from build123d import *

# Parameters (mm, degrees)
SKETCH1_W                    = 117.475
SKETCH1_H                    = 65.3161
BASE_FLANGE1_DEPTH           = 3.2639
F_10_0_1935_DIAMETER_HOLE1_D = 4.9149
BOSS_EXTRUDE1_DEPTH          = 3.2639
F_1_4_START                  = -3.2639
F_1_4_CLEARANCE_SLOT1_DEPTH  = 3.2639
F_10_0_1935_DIAMETER_HOLE2_D = 4.9149
FILLET1_R                    = 6.35
FILLET2_R                    = 12.7


# Read off the part's stored shape, not the designer's step: 1/4 Clearance Slot1
# Sheet-metal steps are written as plain solids
with BuildPart() as part:
    # Sketch1 → Base-Flange1 (new body)
    with BuildSketch(Plane.XY):
        with Locations((58.7375, 0)):
            Rectangle(SKETCH1_W, SKETCH1_H)
    extrude(amount=-BASE_FLANGE1_DEPTH)

    # #10 (0.1935) Diameter Hole1 (through all)
    with Locations(Plane.XY):
        with Locations((28.575, 19.05), (28.575, -19.05), (104.775, 19.05), (104.775, -19.05)):
            Hole(F_10_0_1935_DIAMETER_HOLE1_D / 2)

    # Sketch8 → Boss-Extrude1 (add)
    with BuildSketch(Plane.XY):
        Polygon((0, 32.65805), (-116.888396133, -111.687098016), (-55.202435442, -161.639404056), (49.244605652, -32.65805), (0, -32.65805), align=None)
    extrude(amount=-BOSS_EXTRUDE1_DEPTH)

    # 1/4 Clearance Slot1 outline → 1/4 Clearance Slot1 (cut)
    with BuildSketch(Plane.XY.offset(F_1_4_START)):
        with BuildLine():
            Line((-71.825899608, -91.951886399), (-67.506895384, -95.449347058))
            ThreePointArc((-67.506895384, -95.449347058), (-62.484066487, -94.921426468), (-63.011987077, -89.898597571))
            Line((-63.011987077, -89.898597571), (-67.330991301, -86.401136912))
            ThreePointArc((-67.330991301, -86.401136912), (-72.353820198, -86.929057502), (-71.825899608, -91.951886399))
        make_face()
        with BuildLine():
            ThreePointArc((-42.832511108, -115.430269474), (-37.809682211, -114.902348884), (-38.337602801, -109.879519987))
            Line((-38.337602801, -109.879519987), (-42.656607025, -106.382059328))
            ThreePointArc((-42.656607025, -106.382059328), (-47.679435921, -106.909979918), (-47.151515331, -111.932808814))
            Line((-47.151515331, -111.932808814), (-42.832511108, -115.430269474))
        make_face()
    extrude(amount=F_1_4_CLEARANCE_SLOT1_DEPTH, mode=Mode.SUBTRACT)

    # #10 (0.1935) Diameter Hole2 (through all)
    with Locations(Plane.XY):
        with Locations((-30.326764214, -22.450322184), (-104.256177153, -113.745544006), (14.087127483, -58.415982533), (-59.842285455, -149.711204355), (-6.269239545, -41.93172154), (-80.198652483, -133.226943362), (-8.347749557, 4.69150052)):
            Hole(F_10_0_1935_DIAMETER_HOLE2_D / 2)

    # Fillet1
    fillet1_edges = [part.edges().sort_by_distance(p)[0] for p in [
        (-116.888396133, -111.687098016, -1.63195),
        (-55.202435442, -161.639404056, -1.63195),
        (0, 32.65805, -1.63195),
        (117.475, 32.65805, -1.63195),
        (117.475, -32.65805, -1.63195),
    ]]
    fillet(fillet1_edges, radius=FILLET1_R)

    # Fillet2
    fillet2_edges = [part.edges().sort_by_distance(p)[0] for p in [
        (49.244605652, -32.65805, -1.63195),
    ]]
    fillet(fillet2_edges, radius=FILLET2_R)


solid = part.part
Work out the finished part from the listing and answer in its coordinate system (mm). Round coordinates to 2 decimals unless told otherwise and drop trailing zeros. Write each loop counter-clockwise with the first axis right and the second up, starting at its lowest first coordinate (ties: lowest second). Pieces come first, ordered by that corner, then holes. Notation, with made-up numbers: (-4.75, -12) - (39.25, -12) arc R28 cw to (39.25, 6) - close; hole circle Ø10 at (69, 34.5). An arc over 180 degrees is marked (long way). Answer in a Markdown table with one row per item. Add a question column.
1. A cutting plane is placed at A-A, the plane y = 19.05. Determine the outline of the cut face in (x, z) (3 decimals), and give its area (3 significant figures).
2. Given pin 1 (1 mm diameter, centred on y = -35, z = -0.5, fed in from +X); pin 2 (1 mm diameter, centred on y = -80.5, z = -3, fed in from +X), each flat-ended and moving along its own axis, determine where each tip first touches the part or whether it passes through.
3. A cutting plane is placed at B-B, the plane z = -1.8. Count the separate pieces of the cut face and the enclosed holes in it, and give its area (3 significant figures).
4. Find the intervals of material crossed by line 1 along Y through (x, z) = (107, -2.1); line 2 along X through (y, z) = (-115, -0.3); line 3 along X through (y, z) = (-112, -1.9), in increasing order. Write a range as from..to.
5. A cutting plane is placed at C-C, the plane x = 67. Determine the outline of the cut face in (y, z).
6. A cutting plane is placed at D-D, the plane y = -12. Determine the outline of the cut face in (x, z) (3 decimals).
7. The mould has two halves that part along X. Classify faces 1 (the cylindrical face through (26.305, 18.109, -1.655)), 2 (the flat face through (-86.41, -136.37, -1.61)), 3 (the cylindrical face through (115.66, -30.75, -1.65)): +X half, -X half, draft (parallel to the pull), parting line (faces both ways), or undercut.
Worked out:
| question | item | result |
|---|---|---|
| 1 | outline | (-11.02, -3.264) - (26.118, -3.264) - (26.118, 0) - (-11.02, 0) - close; (31.032, -3.264) - (102.318, -3.264) - (102.318, 0) - (31.032, 0) - close; (107.232, -3.264) - (117.475, -3.264) - (117.475, 0) - (107.232, 0) - close |
| 1 | area | 387 mm^2 |
| 2 | pin 1 | x = 48.71 |
| 2 | pin 2 | x = 10.91 |
| 3 | separate pieces | 1 |
| 3 | enclosed holes | 13 |
| 3 | area | 19,600 mm^2 |
| 4 | line 1 | -32.66..-20.09, -18.01..18.01, 20.09..32.66 |
| 4 | line 2 | -112.67..-106.37, -102.14..-43.36, -37.89..-17.43 |
| 4 | line 3 | -114.18..-105.99, -102.53..-47.07, -37.07..-15.01 |
| 5 | outline | (-32.66, -3.26) - (32.66, -3.26) - (32.66, 0) - (-32.66, 0) - close |
| 6 | outline | (-36.163, -3.264) - (117.475, -3.264) - (117.475, 0) - (-36.163, 0) - close |
| 7 | face 1 | undercut |
| 7 | face 2 | -X half |
| 7 | face 3 | +X half |
